Answer from the drawing. Dimensions are ordinates in mm from the lowest x, y and z of the part. A direction names the side the tool comes from. Give positions to 0.01 mm unless a question says otherwise; leave off trailing zeros. Order: outer loops, then holes, each group sorted by start corner. A loop starts at its lowest first (then second) coordinate and runs counter-clockwise, first axis right, second up.
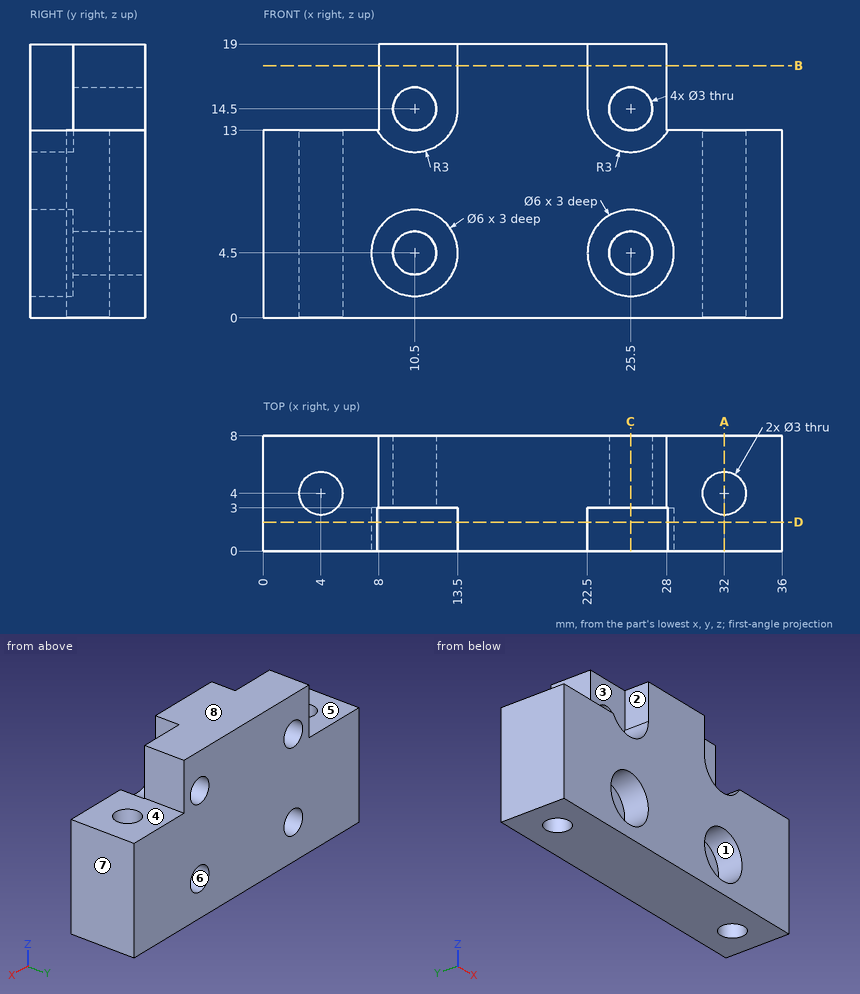
1) The part is cut by section C-C on x = 25.5. Determine the outline of the cut face in (y, z), and give its area (3 significant figures).
Final values:
outline: (0, 0) - (8, 0) - (8, 3) - (3, 3) - (3, 1.5) - (0, 1.5) - close; (0, 7.5) - (3, 7.5) - (3, 6) - (8, 6) - (8, 13) - (3, 13) - (3, 11.5) - (0, 11.5) - close; (3, 16) - (8, 16) - (8, 19) - (3, 19) - close
area: 81.5 mm2
2) For a pull along X with two mould halves and no side action, classify the marked faces 6, 7 and 8 as released by +X, released by -X, zero draft, split by the parting line, or undercut.
Final values:
face 6: undercut
face 7: released by +X
face 8: zero draft
3) Consider L1, parallel to Z at x = 10.5, y = 5.75; L2, parallel to X at y = 5.85, z = 14.5; L3, parallel to X at y = 3.5, z = 9.25. Determine where each line is inside the solid, lowest interval first.
Final values:
L1: z = 0 to 3, 6 to 13, 16 to 19
L2: x = 8 to 9, 12 to 24, 27 to 28
L3: x = 0 to 2.59, 5.41 to 30.59, 33.41 to 36
4) Given pin 1 (2.5 mm diameter, centred on x = 32, y = 4, fed in from +Z); pin 2 (5 mm diameter, centred on x = 10.5, z = 4.5, fed in from -Y); pin 3 (0.9 mm diameter, centred on y = 1, z = 17, fed in from +X); pin 4 (1 mm diameter, centred on x = 6, y = 5, fed in from +Z), each flat-ended and moving along its own axis, determine where each tip first touches the part or whether it passes through.
Final values:
pin 1: passes through
pin 2: stops at y = 3
pin 3: stops at x = 22.5
pin 4: stops at z = 13
5) The part is cut by section A-A on x = 32. Determine the outline of the cut face in (y, z), and give its area (3 significant figures).
Final values:
outline: (0, 0) - (2.5, 0) - (2.5, 13) - (0, 13) - close; (5.5, 0) - (8, 0) - (8, 13) - (5.5, 13) - close
area: 65.0 mm2
6) The part is cut by section B-B on z = 17.5. Determine the outline of the cut face in (x, y).
Final values:
outline: (8, 3) - (13.5, 3) - (13.5, 0) - (22.5, 0) - (22.5, 3) - (28, 3) - (28, 8) - (8, 8) - close
7) The part is cut by section D-D on y = 2. Determine the outline of the cut face in (x, z).
Final values:
outline: (0, 0) - (36, 0) - (36, 13) - (28.1, 13) arc R3 cw to (22.5, 14.5) - (22.5, 19) - (13.5, 19) - (13.5, 14.5) arc R3 cw to (7.9, 13) - (0, 13) - close; hole circle Ø6 at (10.5, 4.5); hole circle Ø6 at (25.5, 4.5)
8) A tool of negligible diameter and unlimited length cuts with its end or side. For the marked faces 1, 2, 3, 4 and 5, from which of +Z, -Z, +X, -X, +Y, -Y can it reach the whole face along a straight path? Write none if from no direction.
Final values:
face 1: -Y
face 2: +Z, -X, -Y
face 3: +Z, -Y
face 4: +Z, +X, +Y, -Y
face 5: +Z, -X, +Y, -Y
